from build123d import *

# Parameters (mm, degrees)
PAD_DEPTH = 30
FILLET_R  = 0.5


with BuildPart() as part:
    # Sketch → Pad (new body)
    with BuildSketch(Plane.XY):
        Polygon((-1.4, 1.4), (-1.4, -14.6), (0, -14.6), (0, 0), (16.4, 0), (16.4, -14.6), (17.8, -14.6), (17.8, 1.4), align=None)
    extrude(amount=PAD_DEPTH)

    # Fillet
    fillet_edges = [part.edges().sort_by_distance(p)[0] for p in [
        (17.8, -6.6, 30),
        (17.1, -14.6, 30),
        (16.4, -7.3, 30),
        (8.2, 0, 30),
        (8.2, 1.4, 30),
        (-1.4, -6.6, 30),
        (0, -7.3, 30),
        (-1.4, 1.4, 15),
        (17.8, 1.4, 15),
        (17.8, -14.6, 15),
        (16.4, -14.6, 15),
        (0, -14.6, 15),
        (-1.4, -14.6, 15),
        (-0.7, -14.6, 30),
        (17.8, -6.6, 0),
        (16.4, -7.3, 0),
        (0, -7.3, 0),
        (-1.4, -6.6, 0),
        (8.2, 1.4, 0),
        (8.2, 0, 0),
    ]]
    fillet(fillet_edges, radius=FILLET_R)


solid = part.part
Design review of the part built by this model. Coordinates are the model's own, in mm. A direction names the side the tool comes from. Round coordinates to 2 decimals unless told otherwise and drop trailing zeros. Loops run counter-clockwise (first coordinate to the right, second up) from the corner with the lowest first, then second, coordinate; pieces in that order, holes last. Notation, with made-up numbers: M 11,14 L 60,14 A13 cw 60,39 Z; hole C -27.75,72.25 d10. An arc over 180 degrees is marked long. Answer as a JSON object with one key per item and string values.
Item 1: We need section C-C on x = 8.5. Give the boundary of the cut face in (y, z), and give its area (3 significant figures).
Answer sheet:
{"outline": "M 0,0.5 A0.5 ccw 0.5,0 L 0.9,0 A0.5 ccw 1.4,0.5 L 1.4,29.5 A0.5 ccw 0.9,30 L 0.5,30 A0.5 ccw 0,29.5 Z", "area": "41.8 mm^2"}
Item 2: We need section B-B on z = 17.5. Give the boundary of the cut face in (x, y), and give its area (3 significant figures).
Answer sheet:
{"outline": "M -1.4,-14.1 A0.5 ccw -0.9,-14.6 L -0.5,-14.6 A0.5 ccw 0,-14.1 L 0,0 L 16.4,0 L 16.4,-14.1 A0.5 ccw 16.9,-14.6 L 17.3,-14.6 A0.5 ccw 17.8,-14.1 L 17.8,0.9 A0.5 ccw 17.3,1.4 L -0.9,1.4 A0.5 ccw -1.4,0.9 Z", "area": "67.4 mm^2"}
Item 3: Wall thickness on L1, parallel to X at y = -10.5, z = 7.25; L2, parallel to Y at x = 1.75, z = 7.5; L3, parallel to Z at x = -0.25, y = -4: over which ranges is each line inside the solid? List them lowest first. Write a range as from..to.
Answer sheet:
{"L1": "x = -1.4..0, 16.4..17.8", "L2": "y = 0..1.4", "L3": "z = 0.07..29.93"}
Item 4: We need section A-A on y = -11.25. Give the boundary of the cut face in (x, z).
Answer sheet:
{"outline": "M -1.4,0.5 A0.5 ccw -0.9,0 L -0.5,0 A0.5 ccw 0,0.5 L 0,29.5 A0.5 ccw -0.5,30 L -0.9,30 A0.5 ccw -1.4,29.5 Z; M 16.4,0.5 A0.5 ccw 16.9,0 L 17.3,0 A0.5 ccw 17.8,0.5 L 17.8,29.5 A0.5 ccw 17.3,30 L 16.9,30 A0.5 ccw 16.4,29.5 Z"}
Item 5: Clearance check with flat-ended pins moving along their axes: P1, Ø8, axis at x = 13.5, y = -7, coming from the -Z side; P2, Ø3, axis at x = 4.5, z = 22, coming from the -Y side; P3, Ø3, axis at x = 13, y = -3.5, coming from the +Z side. State where each tip first meets the part, or that it passes through.
Answer sheet:
{"P1": "stops at z = 0", "P2": "stops at y = 0", "P3": "passes through"}
Item 6: Machinability: for faces 1 (the flat face through (8.2, 0.7, 30)), 2 (the flat face through (16.4, -7, 15)), which of the approach directions +Z, -Z, +X, -X, +Y, -Y give a long, thin tool a straight path to every point of the face, cutting with its end or side? Answer none if there is none.
Answer sheet:
{"face 1": "+Z, +X, -X, +Y, -Y", "face 2": "+Z, -Z, -Y"}
Item 7: The part is to be moulded in two halves that separate along X. For faces 3 (the flat face through (0, -7, 15)), 4 (the flat face through (8, 0, 15)), 5 (the flat face through (17.8, -7, 15)), 6 (the flat face through (-1.4, -6, 15)), say which applies: pulls with the +X half, pulls with the -X half, needs draft (parallel to the pull), parting line crosses it, or undercut.
Answer sheet:
{"face 3": "undercut", "face 4": "undercut", "face 5": "pulls with the +X half", "face 6": "pulls with the -X half"}
